Read the model definition and answer for the solid it produces. Units are mm, in the model's axes. A direction names the side the tool comes from. Coordinates: 2 decimals unless noted, no trailing zeros. Loops run counter-clockwise (first coordinate to the right, second up) from the corner with the lowest first, then second, coordinate; pieces in that order, holes last. Notation, with made-up numbers: (58.25, -10) -> (94.25, -10) arc R21 ccw to (94.25, 14) -> close; hole circle Ø5 at (26, 15). An arc over 180 degrees is marked (long way). Answer as CSV lines item,"result".
```python
from build123d import *

# Parameters (mm, degrees)
CUT_EXTRUDE1_DEPTH = 38.90367873
CIRPATTERN1_COUNT  = 8


with BuildPart() as part:
    # Sketch1 → Revolve1 (revolve)
    with BuildSketch(Plane(origin=(0, 0, 0), x_dir=(0, 0, -1), z_dir=(1, 0, 0)), mode=Mode.PRIVATE) as revolve1_sk:
        with BuildLine():
            Line((0, 0), (0, 36))
            Line((0, 36), (-7, 36))
            Line((-7, 36), (-7, 87.5))
            Line((-7, 87.5), (-51.90367873, 87.5))
            Line((-51.90367873, 87.5), (-51.90367873, 81.59632127))
            ThreePointArc((-51.90367873, 81.59632127), (-56.03239564, 71.62871691), (-66, 67.5))
            Line((-66, 67.5), (-69, 67.5))
            Line((-69, 67.5), (-69, 65.5))
            Line((-69, 65.5), (-11, 65.5))
            Line((-11, 65.5), (-11, 36))
            Line((-11, 36), (-38.057788399, 36))
            Line((-38.057788399, 36), (-55.3, 31.379963326))
            Line((-55.3, 31.379963326), (-55.3, 0))
            Line((-55.3, 0), (0, 0))
        make_face()
    revolve(revolve1_sk.sketch.rotate(Axis((0, 0, 0), (0, 0, -1)), 90), axis=Axis((0, 0, 0), (0, 0, -1)))

    # Sketch2 → Cut-Extrude1 (cut)
    with BuildSketch(Plane.XY.offset(11)):
        with BuildLine():
            Line((75.568573924, 58), (57.393027841, 58))
            ThreePointArc((57.393027841, 58), (32.84389058, 52.485045903), (13.012395116, 37))
            Line((13.012395116, 37), (-15.118999196, 37))
            ThreePointArc((-15.118999196, 37), (-10.556616441, 61.348122111), (3.84175649, 81.505831398))
            Line((3.84175649, 81.505831398), (17.348819511, 93.667645569))
            Line((17.348819511, 93.667645569), (75.568573924, 58))
        make_face()
    cut_extrude1 = extrude(amount=CUT_EXTRUDE1_DEPTH, mode=Mode.SUBTRACT)

    # CirPattern1: Cut-Extrude1 ×8 about axis
    cirpattern1_axis = Axis((0, 0, 0), (0, 0, 1))
    for i in range(1, CIRPATTERN1_COUNT):
        add(cut_extrude1.rotate(cirpattern1_axis, i * 360 / CIRPATTERN1_COUNT), mode=Mode.SUBTRACT)

    # Sketch3 → Revolve2 (revolve)
    with BuildSketch(Plane(origin=(0, 0, 0), x_dir=(0, 0, -1), z_dir=(1, 0, 0))):
        Polygon((5.8, -29.649658317), (5.8, -53), (4.8, -54), (4.8, -127.307937006), (2.8, -127.307937006), (2.8, -29.649658317), align=None)
    revolve(axis=Axis((0, -29.649658317, -2.8), (0, 1, 0)))


solid = part.part
```
Q1. Find the intervals of material crossed by probe 1 along Y at (x, z) = (0, 25); probe 2 along Z at (x, y) = (-52.5, -69); probe 3 along Z at (x, y) = (6.5, -67), in increasing order. Write a range as [from, to].
Results:
probe 1,"y = [-82.02, -77.7], [-36, 36], [77.7, 82.02]"
probe 2,"z = [7, 11], [49.9, 51.9]"
probe 3,"z = [7, 11], [49.9, 69]"
Q2. A cutting plane is placed at C-C, the plane z = 61. Write down the section's boundary in (x, y), and give its area (3 significant figures).
Results:
outline,"circle Ø136.83 at (0, 0); hole circle Ø131 at (0, 0)"
area,"1,230 mm²"
Q3. A cutting plane is placed at A-A, the plane z = 30.5. Give the number of separate pieces and of enclosed holes in the cut face, and give its area (3 significant figures).
Results:
separate pieces,"9"
enclosed holes,"0"
area,"4,780 mm²"
Q4. Given pin 1 Ø4.5 at (x, z) = (0, -3) entering from +Y; pin 2 Ø10 at (x, y) = (-12.5, -9) entering from -Z; pin 3 Ø9 at (x, z) = (60.5, 39) entering from +Y, each flat-ended and moving along its own axis, determine where each tip first touches the part or whether it passes through.
Results:
pin 1,"stops at y = -29.65"
pin 2,"stops at z = 0"
pin 3,"stops at y = 58"
Q5. For a pull along X with two mould halves and no side action, classify faces 5 (the face through (62, 58, 30)), 6 (the face through (-7.07, 73.63, 30.18)), 7 (the face through (73.63, 7.07, 30.18)) as pulls with the +X half, pulls with the -X half, needs draft (parallel to the pull), parting line crosses it, or undercut.
Results:
face 5,"needs draft"
face 6,"undercut"
face 7,"pulls with the +X half"
Q6. For faces 1 (the face through (-39, -72, 51.904)), 2 (the face through (-47.069, -57.064, 30.18)), 3 (the face through (54.484, -49.699, 30.18)), 4 (the face through (-62, -58, 30)), determine the directions among +Z, -Z, +X, -X, +Y, -Y from which every point of the face is accessible in a straight line to the end or side of a thin tool.
Results:
face 1,"+Z"
face 2,"-Y"
face 3,"none"
face 4,"-X, -Y"
